The model under review builds one solid part; all positions refer to its coordinate system, in mm. Face numbers are marked on the shaded views. Give positions to 0.01 mm unless a question says otherwise; leave off trailing zeros. Loops run counter-clockwise (first coordinate to the right, second up) from the corner with the lowest first, then second, coordinate; pieces in that order, holes last. Notation, with made-up numbers: M 25.5,42.25 L 42.5,42.25 A9 ccw 42.5,47.25 Z; hole C 87.5,31 d5. An arc over 180 degrees is marked long. Return JSON: item names as keys, results as strings.
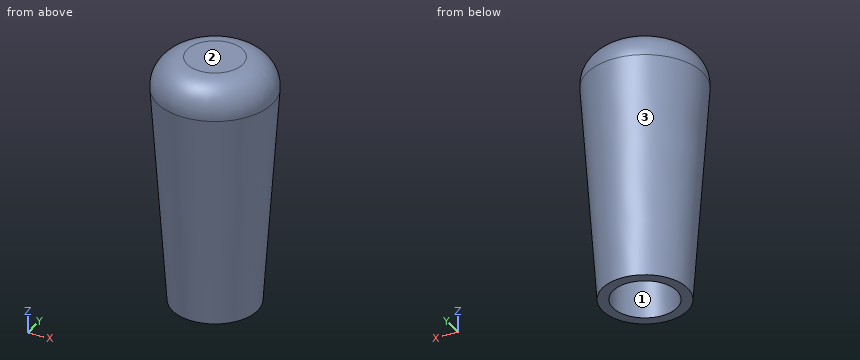
```python
from build123d import *

# Parameters (mm, degrees)
F4_R = 6


with BuildPart() as f1:
    # F0 (on Front) → F1 (revolve)
    with BuildSketch(Plane.XZ):
        Polygon((12, 0), (0, 0), (0, -50), (8.5, -50), align=None)
    revolve(axis=Axis((0, 0, -25), (0, 0, -1)))

    # F2 (on Front) → F3 (revolve, cut)
    with BuildSketch(Plane.XZ):
        Polygon((2.6, -2.013246), (0, -2.013246), (0, -50.013246), (6.4, -50.013246), (5.2, -9.513246), (4, -9.548802), (4, -5.013246), (2.6, -5.013246), align=None)
    revolve(axis=Axis((0, 0, -26.013246), (0, 0, -1)), mode=Mode.SUBTRACT)

    # F4
    f4_edges = [f1.edges().sort_by_distance(p)[0] for p in [
        (-12, 0, 0),
    ]]
    fillet(f4_edges, radius=F4_R)


solid = f1.part
```
1) Consider section A-A on z = -38. Write out the cut boundary in (x, y).
From the geometry:
{"outline": "C 0,0 d18.68; hole C 0,0 d12.09"}
2) The part is to be moulded in two halves that separate along Y. For the marked faces 1, 2 and 3, say which applies: released by +Y, released by -Y, zero draft, split by the parting line, or undercut.
From the geometry:
{"face 1": "undercut", "face 2": "zero draft", "face 3": "split by the parting line"}
3) Wall thickness on L1, parallel to X at y = 0, z = -6.3; L2, parallel to Y at x = 0, z = -4.1; L3, parallel to X at y = -2.5, z = -27: over which ranges is each line inside the solid? List them lowest first. Write a range as from..to.
From the geometry:
{"L1": "-11.56..-4, 4..11.56", "L2": "-11.26..-2.6, 2.6..11.26", "L3": "-9.8..-5.14, 5.14..9.8"}
4) Consider section B-B on z = -21.5. Write out the cut boundary in (x, y) (3 decimals), then the cut area to 3 significant figures.
From the geometry:
{"outline": "C 0,0 d20.99; hole C 0,0 d11.11", "area": "249 mm²"}
5) Insertion check: pin 1 (6 mm diameter, centred on y = 2, z = -43.5, fed in from +X); pin 2 (4 mm diameter, centred on x = 5, y = 8.5, fed in from +Z); pin 3 (8.5 mm diameter, centred on x = 0, y = 0, fed in from -Z). Each pin has a flat end and moves straight along its axis. Give the tip position at first contact, or say it passes through.
From the geometry:
{"pin 1": "x = 9.12", "pin 2": "z = -0.46", "pin 3": "z = -9.55"}
